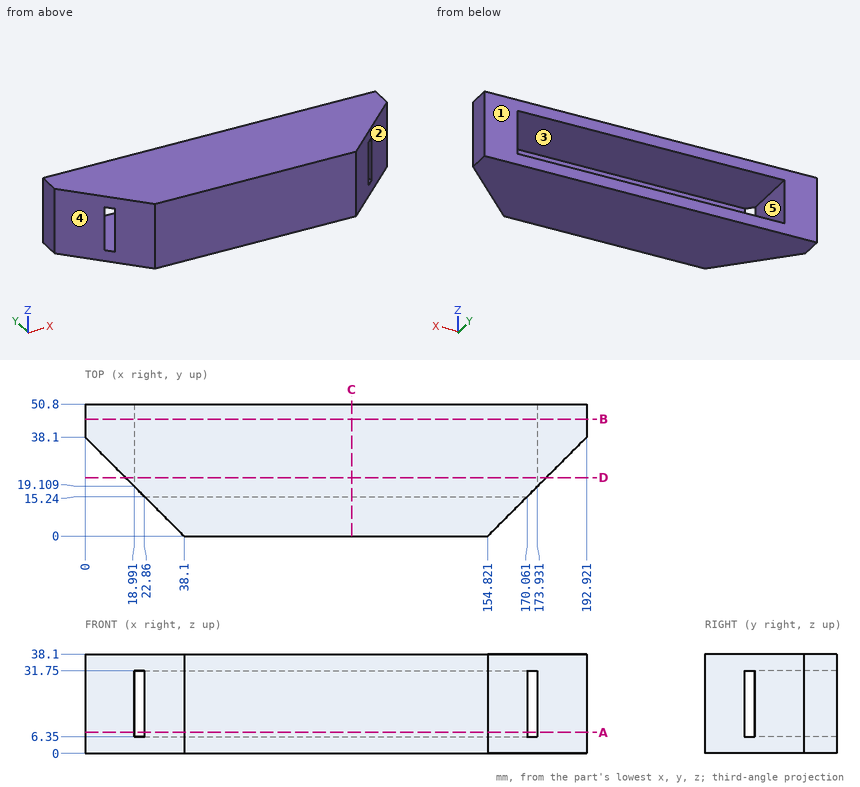
Print and shaded views of the part. All mm, measured from the part's lowest x, y and z. A direction names the side the tool comes from. Round coordinates to 2 decimals unless told otherwise and drop trailing zeros. Write each loop counter-clockwise with the first axis right and the second up, starting at its lowest first coordinate (ties: lowest second). Pieces come first, ordered by that corner, then holes. Notation, with made-up numbers: (38.5, -14) -> (50.5, -14) arc R19 ccw to (50.5, 16) -> close; hole circle Ø4 at (60.5, 46.5). An arc over 180 degrees is marked (long way). Return JSON: item names as keys, results as strings. Group by question number.
Q1. Saw through at A-A on z = 8. Write the cut outline in (x, y), plus the area to 3 significant figures.
Q2. Which spindle directions (+Z, -Z, +X, -X, +Y, -Y) get a long thin tool onto all of the face, cutting with end or side? Do the marked faces 4 and 5. Say none if no direction does.
Q3. Saw through at C-C on x = 102.5. Write the cut outline in (y, z), plus the area to 3 significant figures.
Q4. Saw through at D-D on y = 22.5. Write the cut outline in (x, z).
Q5. Probe L1, parallel to X at y = 41, z = 11; L2, parallel to Z at x = 86.5, y = 30.5; L3, parallel to Y at x = 72.5, z = 27. List the from-to ranges inside material, lowest first. Write a range as [from, to].
Q6. Pin check, flat tips, straight feed: pin 1 (12.5 mm diameter, centred on x = 110, z = 14, fed in from +Y); pin 2 (4 mm diameter, centred on x = 168, z = 31.5, fed in from -Y); pin 3 (12.5 mm diameter, centred on y = 27.5, z = 16.5, fed in from +X). Stop position of each tip, or through.
Q7. Saw through at B-B on y = 45. Write the cut outline in (x, z).
Q8. Mould opens along X. For the marked faces 1, 2 and 3 say: pulls with the +X half, pulls with the -X half, needs draft (parallel to the pull), parting line crosses it, or undercut.
Answer:
{
 "1": {"outline": "(0, 38.1) -> (18.99, 19.11) -> (18.99, 50.8) -> (0, 50.8) -> close; (22.86, 15.24) -> (38.1, 0) -> (154.82, 0) -> (170.06, 15.24) -> close; (173.93, 19.11) -> (192.92, 38.1) -> (192.92, 50.8) -> (173.93, 50.8) -> close", "area": "2,850 mm2"},
 "2": {"face 4": "+Z, -Z, -X, -Y", "face 5": "+Y, -Y"},
 "3": {"outline": "(0, 0) -> (50.8, 0) -> (50.8, 6.35) -> (15.24, 6.35) -> (15.24, 31.75) -> (50.8, 31.75) -> (50.8, 38.1) -> (0, 38.1) -> close", "area": "1,030 mm2"},
 "4": {"outline": "(15.6, 0) -> (177.32, 0) -> (177.32, 38.1) -> (15.6, 38.1) -> close; hole (18.99, 6.35) -> (173.93, 6.35) -> (173.93, 31.75) -> (18.99, 31.75) -> close"},
 "5": {"L1": "[0, 18.99], [173.93, 192.92]", "L2": "[0, 6.35], [31.75, 38.1]", "L3": "[0, 15.24]"},
 "6": {"pin 1": "y = 15.24", "pin 2": "y = 11.18", "pin 3": "x = 188.57"},
 "7": {"outline": "(0, 0) -> (192.92, 0) -> (192.92, 38.1) -> (0, 38.1) -> close; hole (18.99, 6.35) -> (173.93, 6.35) -> (173.93, 31.75) -> (18.99, 31.75) -> close"},
 "8": {"face 1": "needs draft", "face 2": "pulls with the +X half", "face 3": "undercut"}
}
